Work out the finished part from the listing and answer in its coordinate system (mm). A direction names the side the tool comes from. Round coordinates to 2 decimals unless told otherwise and drop trailing zeros. Write each loop counter-clockwise with the first axis right and the second up, starting at its lowest first coordinate (ties: lowest second). Pieces come first, ordered by that corner, then holes. Notation, with made-up numbers: (10.25, 86.5) - (65.25, 86.5) arc R23 ccw to (65.25, 116.5) - close; hole circle Ø11 at (-17.75, 2.5). An arc over 180 degrees is marked (long way). Write item = value, one per line. Start each with the question number.
Autodesk Inventor part; units mm, degrees
ref_plane "YZ Plane" through (0, 0, 0) normal (1, 0, 0) x (0, 1, 0)
ref_plane "XZ Plane" through (0, 0, 0) normal (0, 1, 0) x (-1, 0, 0)
ref_plane "XY Plane" through (0, 0, 0) normal (0, 0, 1) x (1, 0, 0)
sketch "Skizze1" plane through (0, 0, 0) normal (0, 1, 0) x (-1, 0, 0)
  circle A0 centre (0, 0) radius 45
  circle A1 centre (0, 0) radius 35
  dimension "d0" = 90
  dimension "d1" = 70
extrude "Extrusion1" add sketch "Skizze1" along normal blind 3
sketch "Skizze6" plane through (0, 0, 0) normal (0, -1, 0) x (1, 0, 0)
  circle A0 centre (0, 0) radius 35
  line L0 (-36.1127, -36.1127) -> (36.1127, -36.1127) construction
  line L1 (36.1127, -36.1127) -> (36.1127, 36.1127) construction
  line L2 (36.1127, 36.1127) -> (-36.1127, 36.1127) construction
  line L3 (-36.1127, 36.1127) -> (-36.1127, -36.1127) construction
  line L4 (-36.1127, -36.1127) -> (36.1127, 36.1127) construction
  line L5 (36.1127, -36.1127) -> (-36.1127, 36.1127) construction
  circle A1 centre (0, 0) radius 45 construction
  line L6 (-26.1127, 26.1127) -> (-36.1127, 26.1127)
  line L7 (-36.1127, 26.1127) -> (-36.1127, 36.1127)
  line L8 (-36.1127, 36.1127) -> (-26.1127, 36.1127)
  line L9 (-26.1127, 36.1127) -> (-26.1127, 26.1127)
  line L10 (-26.1127, 26.1127) -> (-36.1127, 36.1127) construction
  line L11 (-36.1127, 26.1127) -> (-26.1127, 36.1127) construction
  line L12 (-26.1127, -26.1127) -> (-26.1127, -36.1127)
  line L13 (-26.1127, -36.1127) -> (-36.1127, -36.1127)
  line L14 (-36.1127, -36.1127) -> (-36.1127, -26.1127)
  line L15 (-26.1127, -26.1127) -> (-36.1127, -36.1127) construction
  line L16 (-26.1127, -36.1127) -> (-36.1127, -26.1127) construction
  line L17 (-36.1127, -26.1127) -> (-26.1127, -26.1127)
  line L18 (26.1127, -26.1127) -> (36.1127, -26.1127)
  line L19 (36.1127, -26.1127) -> (36.1127, -36.1127)
  line L20 (36.1127, -36.1127) -> (26.1127, -36.1127)
  line L21 (26.1127, -26.1127) -> (36.1127, -36.1127) construction
  line L22 (36.1127, -26.1127) -> (26.1127, -36.1127) construction
  line L23 (26.1127, -36.1127) -> (26.1127, -26.1127)
  line L24 (26.1127, 26.1127) -> (26.1127, 36.1127)
  line L25 (26.1127, 36.1127) -> (36.1127, 36.1127)
  line L26 (36.1127, 36.1127) -> (36.1127, 26.1127)
  line L27 (26.1127, 26.1127) -> (36.1127, 36.1127) construction
  line L28 (26.1127, 36.1127) -> (36.1127, 26.1127) construction
  line L29 (36.1127, 26.1127) -> (26.1127, 26.1127)
  point P0 (-31.1127, 31.1127)
  point P1 (-31.1127, -31.1127)
  point P2 (31.1127, -31.1127)
  point P3 (31.1127, 31.1127)
  dimension "d54" = 44
  dimension "d55" = 10
  dimension "d56" = 10
  dimension "d59" = 360
extrude "Extrusion4" add sketch "Skizze6" against normal blind 3 contours L6 L7 L8 L9 | L12 L13 L14 L17 | L18 L19 L20 L23 | L24 L25 L26 L29
sketch "Skizze7" plane through (0, 3, 0) normal (0, 1, 0) x (1, 0, 0)
  line L0 (-36.1127, -26.8491) -> (-36.1127, -36.1127)
  line L1 (-36.1127, -36.1127) -> (-26.8491, -36.1127)
  point P0 (0, 0)
  point P1 (-32.1127, -32.1127)
  point P2 (32.1127, -32.1127)
  point P3 (32.1127, 32.1127)
  point P4 (-32.1127, 32.1127)
  dimension "d63" = 4
  dimension "d64" = 4
  dimension "d67" = 360
hole "Bohrung3" at (-32.1127, 3, 32.1127) at (32.1127, 3, 32.1127) at (32.1127, 3, -32.1127) at (-32.1127, 3, -32.1127) direction (0, -1, 0) diameter 3.3 end through all
fillet "Rundung1" radius 2 4 edges at (-36.1127, 1.5, 36.1127) (-36.1127, 1.5, -36.1127) (36.1127, 1.5, 36.1127) (36.1127, 1.5, -36.1127)
properties part number "LED_Ring"
1. Which of the six approach directions +Z, -Z, +X, -X, +Y, -Y give full straight-line access (tool end or side, diameter ignored) to faces 1 (the face through (36.113, 1, 31)), 2 (the face through (-30, 1, -36.113)), 3 (the face through (-36.113, 1, 30)), 4 (the face through (31, 1, -36.113))?
2. Each of these flat-tipped pins is pushed along its axis until it touches: pin 1 (1.5 mm diameter, centred on y = 1.5, z = -30, fed in from -X); pin 2 (1.5 mm diameter, centred on y = 1.5, z = 31.5, fed in from +X); pin 3 (1.5 mm diameter, centred on x = 29, y = 1.5, fed in from +Z). Where does it stop, or does it pass through?
3. Find section B-B on x = 0. Give the vertices of the cut face in (y, z).
4. For a pull along Z with two mould halves and no side action, classify faces 5 (the face through (36.113, 1, -30)), 6 (the face through (-45, 1, 0)), 7 (the face through (33.58, 1.48, 32.87)) as released by +Z, released by -Z, zero draft, split by the parting line, or undercut.
5. Find section A-A on z = 0. Give the vertices of the cut face in (x, y).
6. Consider line 1 (X direction, y = 1.1, z = -1); line 2 (Z direction, x = 0, y = 2.35); line 3 (X direction, y = 0.6, z = 32.5). Determine where each line is inside the solid, lowest interval first.
7. Find section C-C on y = 1.65. Give the vertices of the cut face in (x, z).
Answer key:
q1.face_1 = +Z, +X, +Y, -Y
q1.face_2 = -Z, -X, +Y, -Y
q1.face_3 = +Z, -X, +Y, -Y
q1.face_4 = -Z, +X, +Y, -Y
q2.pin_1 = -36.11
q2.pin_2 = 36.11
q2.pin_3 = 36.11
q3.outline = (0, -45) - (3, -45) - (3, -35) - (0, -35) - close; (0, 35) - (3, 35) - (3, 45) - (0, 45) - close
q4.face_5 = zero draft
q4.face_6 = split by the parting line
q4.face_7 = undercut
q5.outline = (-45, 0) - (-35, 0) - (-35, 3) - (-45, 3) - close; (35, 0) - (45, 0) - (45, 3) - (35, 3) - close
q6.line_1 = -44.99 to -34.99, 34.99 to 44.99
q6.line_2 = -45 to -35, 35 to 45
q6.line_3 = -36.11 to -33.72, -30.51 to -12.99, 12.99 to 30.51, 33.72 to 36.11
q7.outline = (-36.11, -34.11) arc R2 ccw to (-34.11, -36.11) - (-26.85, -36.11) arc R45 ccw to (26.85, -36.11) - (34.11, -36.11) arc R2 ccw to (36.11, -34.11) - (36.11, -26.85) arc R45 ccw to (36.11, 26.85) - (36.11, 34.11) arc R2 ccw to (34.11, 36.11) - (26.85, 36.11) arc R45 ccw to (-26.85, 36.11) - (-34.11, 36.11) arc R2 ccw to (-36.11, 34.11) - (-36.11, 26.85) arc R45 ccw to (-36.11, -26.85) - close; hole circle Ø70 at (0, 0); hole circle Ø3.3 at (-32.11, -32.11); hole circle Ø3.3 at (-32.11, 32.11); hole circle Ø3.3 at (32.11, -32.11); hole circle Ø3.3 at (32.11, 32.11)
